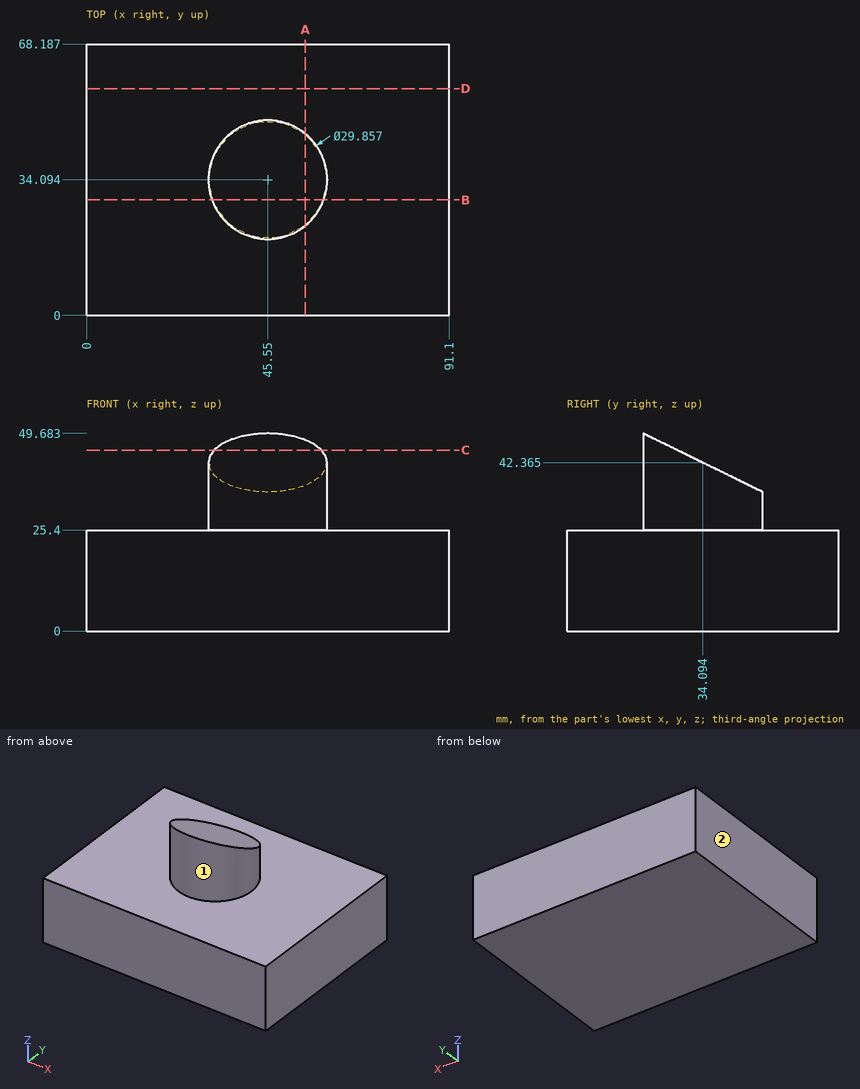
Design review of the part shown in the three views and the two pictorial views. Dimensions are in mm from the part's minimum x, y and z. A direction names the side the tool comes from. Round coordinates to 2 decimals unless told otherwise and drop trailing zeros. Write each loop counter-clockwise with the first axis right and the second up, starting at its lowest first coordinate (ties: lowest second). Pieces come first, ordered by that corner, then holes. Notation, with made-up numbers: (-13, -29) -> (3, -29) arc R16 ccw to (3, -3) -> close; hole circle Ø3 at (86.25, 41.5). An arc over 180 degrees is marked (long way). Write item = value, one per line. Start each with the question number.
1) Wall thickness on probe 1 along Z at (x, y) = (22, 50); probe 2 along Y at (x, z) = (45.5, 26) (1 decimal); probe 3 along Z at (x, y) = (45, 41.5) (1 decimal): over which ranges is each line inside the solid? List them lowest first. Write a range as from..to.
2) Take a section at D-D, the plane y = 57. State the section outline as (x, z) points, plus the area to 3 significant figures.
3) Take a section at C-C, the plane z = 45.5. State the section outline as (x, y) points, plus the area to 3 significant figures.
4) Take a section at A-A, the plane x = 55. State the section outline as (y, z) points.
5) Take a section at B-B, the plane y = 29. State the section outline as (x, z) points, plus the area to 3 significant figures.
6) Tool access review of the marked faces 1 and 2: name each direction out of +Z, -Z, +X, -X, +Y, -Y from which nothing blocks a thin tool from reaching the whole face with its end or side.
7) Clearance check with flat-ended pins moving along their axes: pin 1 (12 mm diameter, centred on x = 34, z = 44.5, fed in from -Y) (1 decimal); pin 2 (1 mm diameter, centred on x = 47, y = 55.5, fed in from +Z); pin 3 (3 mm diameter, centred on y = 38, z = 34, fed in from -X). State where each tip first meets the part, or that it passes through.
Results list:
q1.probe_1 = 0..25.4
q1.probe_2 = 19.2..49
q1.probe_3 = 0..38.7
q2.outline = (0, 0) -> (91.1, 0) -> (91.1, 25.4) -> (0, 25.4) -> close
q2.area = 2,310 mm²
q3.outline = (32.06, 27.7) arc R14.93 ccw to (59.04, 27.7) -> close
q3.area = 165 mm²
q4.outline = (0, 0) -> (68.19, 0) -> (68.19, 25.4) -> (45.65, 25.4) -> (45.65, 36.7) -> (22.54, 48.03) -> (22.54, 25.4) -> (0, 25.4) -> close
q5.outline = (0, 0) -> (91.1, 0) -> (91.1, 25.4) -> (59.58, 25.4) -> (59.58, 44.86) -> (31.52, 44.86) -> (31.52, 25.4) -> (0, 25.4) -> close
q5.area = 2,860 mm²
q6.face_1 = +Z
q6.face_2 = +Z, -Z, -X, +Y, -Y
q7.pin_1 = 20.2
q7.pin_2 = 25.4
q7.pin_3 = 30.82
